Autodesk Fusion 360 part; units mm, degrees
sketch "스케치1" plane through (0, 0, 0) normal (0, 1, 0) x (1, 0, 0)
  circle A0 centre (0, 0) radius 12.15
  circle A1 centre (11.15, 0) radius 4.9
  circle A2 centre (-11.15, 0) radius 4.9
  circle A3 centre (13.35, 0) radius 1.3
  circle A4 centre (-13.35, 0) radius 1.3
  circle A5 centre (13.35, 0) radius 1.925
  circle A6 centre (-13.35, 0) radius 1.925
  dimension "d1" = 24.3
  dimension "d2" = 9.8
  dimension "d3" = 9.8
  dimension "d4" = 2.6
  dimension "d5" = 2.2
  dimension "d6" = 2.6
  dimension "d7" = 2.2
  dimension "d8" = 11.15
  dimension "d9" = 11.15
  dimension "d10" = 3.85
  dimension "d11" = 3.85
extrude "돌출1" add sketch "스케치1" along normal blind 2.2
extrude "돌출2" cut sketch "스케치1" along normal blind 1.6 contours A0 A4 A6 | A0 A4 A6 | A0 A4 | A0 A4
extrude "돌출3" cut sketch "스케치1" along normal blind 1.6 contours A0 A3 | A0 A3 A5 | A0 A3 A5 picked at (13.8121, -0.0629)
extrude "돌출4" cut sketch "스케치1" along normal blind 2.2 contours A0 A3 | A0 A3
extrude "돌출5" cut sketch "스케치1" along normal blind 2.2 contours A0 A4 | A0 A4
sketch "스케치2" plane through (0, 2.2, 0) normal (0, 1, 0) x (-1, 0, 0)
  circle A0 centre (13.35, 0) radius 1.3
  circle A1 centre (-13.35, 0) radius 1.3
  arc A2 (-11.1182, -4.8999) -> (11.1182, -4.8999) centre (0, 0) ccw
  arc A3 (11.1182, -4.8999) -> (11.1182, 4.8999) centre (11.15, 0) ccw
  arc A4 (11.1182, 4.8999) -> (-11.1182, 4.8999) centre (0, 0) ccw
  arc A5 (-11.1182, 4.8999) -> (-11.1182, -4.8999) centre (-11.15, 0) ccw
  circle A6 centre (0, 0) radius 10.25
  circle A7 centre (0, 0) radius 9.15
  dimension "d22" = 20.5
  dimension "d23" = 18.3
extrude "돌출6" add sketch "스케치2" along normal blind 1.5 contours A6
sketch "스케치3" plane through (0, 2.2, 0) normal (0, 1, 0) x (-1, 0, 0)
  circle A0 centre (0, 0) radius 9.15
  line L0 (3, -7.86) -> (-3, -7.86)
  line L1 (-4.6, -6.26) -> (-4.6, -6.2)
  line L2 (-3, -4.6) -> (3, -4.6)
  line L3 (4.6, -6.2) -> (4.6, -6.26)
  arc A1 (-4.6, -6.26) -> (-3, -7.86) centre (-3, -6.26) ccw
  arc A2 (-3, -4.6) -> (-4.6, -6.2) centre (-3, -6.2) ccw
  arc A3 (3, -7.86) -> (4.6, -6.26) centre (3, -6.26) ccw
  arc A4 (4.6, -6.2) -> (3, -4.6) centre (3, -6.2) ccw
  point P0 (4.6, -7.86)
  point P1 (-4.6, -7.86)
  point P2 (4.6, -4.6)
  point P3 (0, -4.6)
  dimension "d26" = 9.2
  dimension "d27" = 3.26
  dimension "d28" = 1.6
  dimension "d29" = 1.6
  dimension "d30" = 1.6
  dimension "d31" = 1.6
  dimension "d32" = 4.6
extrude "돌출7" cut sketch "스케치3" against normal blind 10 contours L0 L1 L2 L3 A1 A2 A3 A4
Geometry: final body of the model. Coordinates: model frame, mm. A direction names the side the tool comes from. Coordinates: 2 decimals unless noted, no trailing zeros. Order: outer loops, then holes, each group sorted by start corner. A loop starts at its lowest first (then second) coordinate and runs counter-clockwise, first axis right, second up.
1) Ray query, probe 1 along X at (y, z) = (1.25, 0) (3 decimals); probe 2 along Z at (x, y) = (0, 2.95); probe 3 along Z at (x, y) = (-13.35, 0.5) (3 decimals). Return the intervals inside material, ascending.
Result sheet:
probe 1: x = -16.05 to -15.275, -11.425 to 11.425, 15.275 to 16.05
probe 2: z = -10.25 to -9.15, 9.15 to 10.25
probe 3: z = -4.378 to -1.925, 1.925 to 4.378
2) Section C-C (x = 0). Return loops of the section in (y, z).
Result sheet:
outline: (0, -12.15) - (2.2, -12.15) - (2.2, -10.25) - (3.7, -10.25) - (3.7, -9.15) - (2.2, -9.15) - (2.2, -7.86) - (0, -7.86) - close; (0, -4.6) - (2.2, -4.6) - (2.2, 9.15) - (3.7, 9.15) - (3.7, 10.25) - (2.2, 10.25) - (2.2, 12.15) - (0, 12.15) - close
3) Section A-A (z = 0). Return loops of the section in (x, y) (3 decimals), then the cut area to 3 significant figures.
Result sheet:
outline: (-16.05, 0) - (-15.275, 0) - (-15.275, 1.6) - (-14.65, 1.6) - (-14.65, 2.2) - (-16.05, 2.2) - close; (-12.05, 1.6) - (-11.425, 1.6) - (-11.425, 0) - (11.425, 0) - (11.425, 1.6) - (12.05, 1.6) - (12.05, 2.2) - (10.25, 2.2) - (10.25, 3.7) - (9.15, 3.7) - (9.15, 2.2) - (-9.15, 2.2) - (-9.15, 3.7) - (-10.25, 3.7) - (-10.25, 2.2) - (-12.05, 2.2) - close; (14.65, 1.6) - (15.275, 1.6) - (15.275, 0) - (16.05, 0) - (16.05, 2.2) - (14.65, 2.2) - close
area: 58.5 mm2
4) First-contact query: P1, Ø11, axis at x = 0, z = 0, coming from the +Y side; P2, Ø1, axis at y = 1.5, z = -8.5, coming from the -X side; P3, Ø2, axis at x = -13.35, z = 0, coming from the -Y side; P4, Ø1, axis at x = 9, y = 3, coming from the +Z side. Flat tips, straight axial feed; report the tip coordinate or a pass-through.
Result sheet:
P1: stops at y = 2.2
P2: stops at x = -9.14
P3: passes through
P4: stops at z = 5.73
5) Section D-D (y = 2.85). Return loops of the section in (x, z).
Result sheet:
outline: circle Ø20.5 at (0, 0); hole circle Ø18.3 at (0, 0)
6) Set-up query: faces 4 (the cylindrical face through (11.427, 0.789, 0.085)), 5 (the flat face through (0, 2.2, 0)), 6 (the cylindrical face through (0.2, 1.08, 12.15)), 7 (the flat face through (0, 1, -4.6)). Return all of +Z, -Z, +X, -X, +Y, -Y with unobstructed straight access to the full face (end or side cutting, diameter ignored); none if empty.
Result sheet:
face 4: -Y
face 5: +Y
face 6: +Z, +Y, -Y
face 7: +Y, -Y
7) Section B-B (y = 1.25). Return loops of the section in (x, z) (3 decimals).
Result sheet:
outline: (-11.118, -4.9) arc R12.15 ccw to (11.118, -4.9) arc R4.9 ccw (long way) to (11.118, 4.9) arc R12.15 ccw to (-11.118, 4.9) arc R4.9 ccw (long way) to start; hole circle Ø3.85 at (-13.35, 0); hole (-4.6, -6.26) arc R1.6 ccw to (-3, -7.86) - (3, -7.86) arc R1.6 ccw to (4.6, -6.26) - (4.6, -6.2) arc R1.6 ccw to (3, -4.6) - (-3, -4.6) arc R1.6 ccw to (-4.6, -6.2) - close; hole circle Ø3.85 at (13.35, 0)
8) Draft query along Z for faces 1 (the cylindrical face through (-12.11, 1.9, 0.39)), 2 (the cylindrical face through (-0.2, 1.08, -12.15)), 3 (the cylindrical face through (-16.05, 1.08, 0.11)). Return one class per face: released by +Z, released by -Z, zero draft, split by the parting line, or undercut.
Result sheet:
face 1: undercut
face 2: released by -Z
face 3: split by the parting line
